Source: three-view drawing plus pictorial views. Frame: mm from the lowest corner of the part. A direction names the side the tool comes from. Round coordinates to 2 decimals unless told otherwise and drop trailing zeros. Loops run counter-clockwise (first coordinate to the right, second up) from the corner with the lowest first, then second, coordinate; pieces in that order, holes last. Notation, with made-up numbers: (47, 85.25) -> (106, 85.25) arc R26 cw to (106, 124.25) -> close; hole circle Ø5 at (-19, 2). An arc over 180 degrees is marked (long way). Put each result on its own line as item: value. Start each with the question number.
1. Draft query along Y for the marked faces 3, 4 and 5. Return one class per face: pulls with the +Y half, pulls with the -Y half, needs draft (parallel to the pull), parting line crosses it, or undercut.
2. Material intervals for L1, parallel to Y at x = 5, z = 5.05; L2, parallel to Z at x = 5, y = 30.5; L3, parallel to Y at x = 5, z = 0.8, sorted ascending.
3. Cut plane B-B (x = 5). Return the cut outline in (y, z), then the cut area to 3 significant figures.
4. Set-up query: the marked faces 1 and 2. Return all of +Z, -Z, +X, -X, +Y, -Y with unobstructed straight access to the full face (end or side cutting, diameter ignored); none if empty.
5. Contact query for flat-ended pins moving along their axis: pin 1 (3 mm diameter, centred on x = 8, y = 15, fed in from -Z); pin 2 (2 mm diameter, centred on y = 16, z = 1, fed in from +X). Output: stop coordinate, or through.
6. Cut plane A-A (y = 20). Return the cut outline in (x, z), then the cut area to 3 significant figures.
7. Cut plane D-D (x = 8). Return the cut outline in (y, z), then the cut area to 3 significant figures.
8. Cut plane C-C (y = 7). Return the cut outline in (x, z).
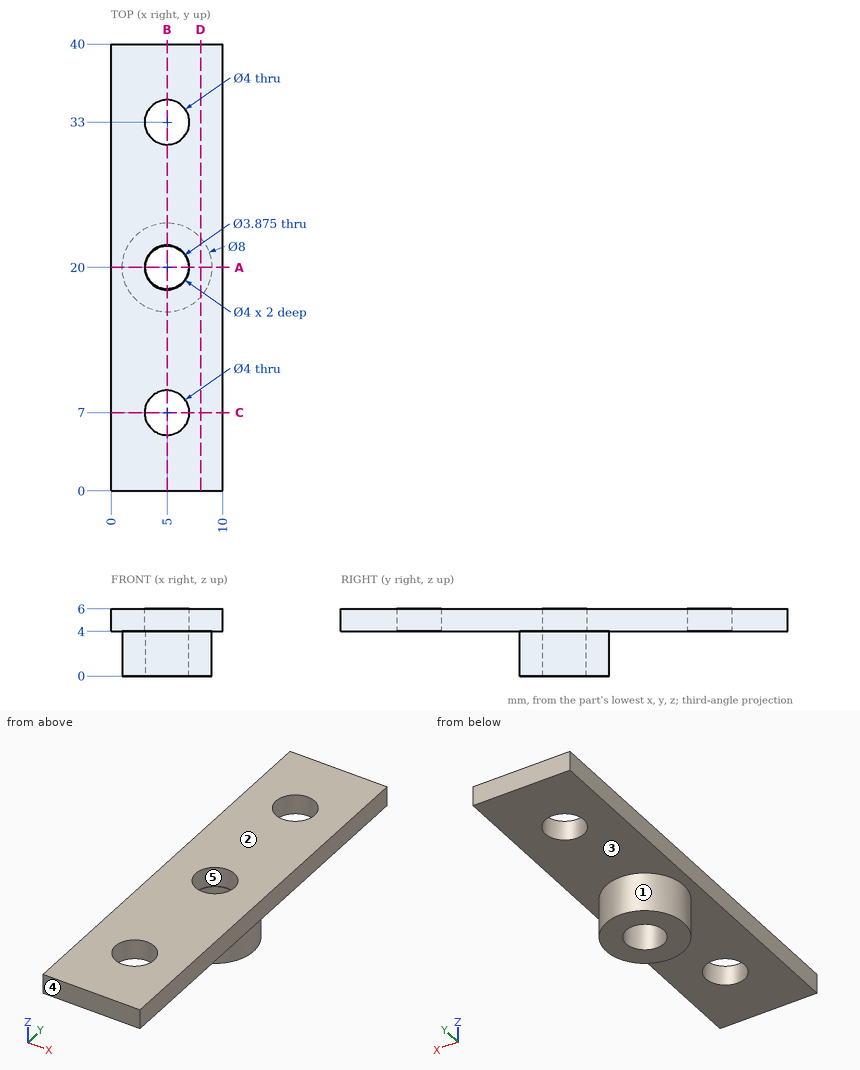
Solution:
1. face 3: needs draft
1. face 4: pulls with the -Y half
1. face 5: undercut
2. L1: y = 0 to 5, 9 to 18, 22 to 31, 35 to 40
2. L2: z = 4 to 6
2. L3: y = 16 to 18.06, 21.94 to 24
3. outline: (0, 4) -> (5, 4) -> (5, 6) -> (0, 6) -> close; (9, 4) -> (16, 4) -> (16, 0) -> (18.06, 0) -> (18.06, 4) -> (18, 4) -> (18, 6) -> (9, 6) -> close; (21.94, 0) -> (24, 0) -> (24, 4) -> (31, 4) -> (31, 6) -> (22, 6) -> (22, 4) -> (21.94, 4) -> close; (35, 4) -> (40, 4) -> (40, 6) -> (35, 6) -> close
3. area: 72.5 mm^2
4. face 1: -Z
4. face 2: +Z, +X, -X, +Y, -Y
5. pin 1: stops at z = 4
5. pin 2: stops at x = 7.65
6. outline: (0, 4) -> (1, 4) -> (1, 0) -> (3.06, 0) -> (3.06, 4) -> (3, 4) -> (3, 6) -> (0, 6) -> close; (6.94, 0) -> (9, 0) -> (9, 4) -> (10, 4) -> (10, 6) -> (7, 6) -> (7, 4) -> (6.94, 4) -> close
6. area: 28.5 mm^2
7. outline: (0, 4) -> (17.35, 4) -> (17.35, 0) -> (22.65, 0) -> (22.65, 4) -> (40, 4) -> (40, 6) -> (0, 6) -> close
7. area: 101 mm^2
8. outline: (0, 4) -> (3, 4) -> (3, 6) -> (0, 6) -> close; (7, 4) -> (10, 4) -> (10, 6) -> (7, 6) -> close
